Source: CAD feature listing. Evaluate the final solid. Frame: model axes, mm. A direction names the side the tool comes from. Round coordinates to 2 decimals unless told otherwise and drop trailing zeros. Write each loop counter-clockwise with the first axis right and the second up, starting at its lowest first coordinate (ties: lowest second). Pieces come first, ordered by that corner, then holes.
from build123d import *

# Parameters (mm, degrees)
F0_W           = 101.6
F0_H           = 203.2
F1_DEPTH       = 25.4
F2_W           = 22.9419407606
F2_H           = 22.7780664682
F2_W_2         = 22.94193331
F2_W_3         = 22.9362
F2_H_2         = 22.6314
F3_DEPTH       = 70.612
F4_W           = 50.8
F4_H           = 203.2
F5_DEPTH       = 9.525
F6_W           = 101.6606390476
F6_H           = 50.6004877388
F7_DEPTH       = 9.525
F8_W           = 50.696041435
F8_H           = 203.55078578
F9_DEPTH       = 9.525
F10_W          = 101.6
F10_H          = 50.8
F11_DEPTH      = 0.762
F11_DEPTH_BACK = 25.4
F12_DEPTH      = 25.4
F13_R          = 12.6564144883
F14_DEPTH      = 33.02


with BuildPart() as f1:
    # F0 (on Front) → F1 (new body)
    with BuildSketch(Plane.XZ):
        Rectangle(F0_W, F0_H)
    extrude(amount=F1_DEPTH)

    # F2 (on face) → F3 (join)
    with BuildSketch(Plane.XZ.offset(25.4)):
        with Locations((39.3290296197, 90.2109667659)):
            Rectangle(F2_W, F2_H)
        with Locations((-39.329033345, 90.2109667659)):
            Rectangle(F2_W_2, F2_H)
        with Locations((-39.3319, -89.9565626328)):
            Rectangle(F2_W_3, F2_H_2)
        with Locations((39.3319, -90.2023647373)):
            Rectangle(F2_W_3, F2_H_2)
    extrude(amount=F3_DEPTH)

    # F4 (on face) → F5 (join)
    with BuildSketch(Plane.YZ.offset(50.8)):
        Rectangle(F4_W, F4_H)
    extrude(amount=F5_DEPTH)

    # F6 (on face) → F7 (join)
    with BuildSketch(Plane.XY.offset(101.6)):
        Rectangle(F6_W, F6_H)
    extrude(amount=F7_DEPTH)

    # F8 (on face) → F9 (join)
    with BuildSketch(Plane(origin=(-50.8, 0, 0), x_dir=(0, -1, 0), z_dir=(-1, 0, 0))):
        Rectangle(F8_W, F8_H)
    extrude(amount=F9_DEPTH)

    # F10 (on face) → F11 (join, two sides)
    with BuildSketch(Plane(origin=(0, 0, -101.6), x_dir=(1, 0, 0), z_dir=(0, 0, -1))) as f11_sk:
        Rectangle(F10_W, F10_H)
    extrude(amount=F11_DEPTH)
    extrude(f11_sk.sketch, amount=-F11_DEPTH_BACK)

    # F2 (on face) → F12 (join)
    with BuildSketch(Plane.XZ.offset(25.4)):
        with Locations((39.3290296197, 90.2109667659)):
            Rectangle(F2_W, F2_H)
        with Locations((-39.329033345, 90.2109667659)):
            Rectangle(F2_W_2, F2_H)
        with Locations((-39.3319, -89.9565626328)):
            Rectangle(F2_W_3, F2_H_2)
        with Locations((39.3319, -90.2023647373)):
            Rectangle(F2_W_3, F2_H_2)
    extrude(amount=F12_DEPTH)

    # F13 (on face) → F14 (join)
    with BuildSketch(Plane.XZ.offset(25.4)):
        Circle(F13_R)
    extrude(amount=-F14_DEPTH)


solid = f1.part
1) Section query B-B on z = 0. Return the cut outline in (x, y) (3 decimals).
Taken from the geometry:
outline: (-60.325, -25.348) - (-50.8, -25.348) - (-50.8, -25.4) - (60.325, -25.4) - (60.325, 25.4) - (50.8, 25.4) - (50.8, 0) - (12.656, 0) - (12.656, 7.62) - (-12.656, 7.62) - (-12.656, 0) - (-50.8, 0) - (-50.8, 25.348) - (-60.325, 25.348) - close
2) Pull-direction query (X, two-part tool) for faces 1 (the face through (-50.83, 0, 106)), 2 (the face through (50.8, -60, -90)), 3 (the face through (-1, 13, 101.6)); classes: released by +X, released by -X, zero draft, split by the parting line, or undercut.
Taken from the geometry:
face 1: released by -X
face 2: released by +X
face 3: undercut
3) Section query A-A on y = -75.5. Return the cut outline in (x, z).
Taken from the geometry:
outline: (-50.8, -101.27) - (-27.86, -101.27) - (-27.86, -78.64) - (-50.8, -78.64) - close; (-50.8, 78.82) - (-27.86, 78.82) - (-27.86, 101.6) - (-50.8, 101.6) - close; (27.86, -101.52) - (50.8, -101.52) - (50.8, -78.89) - (27.86, -78.89) - close; (27.86, 78.82) - (50.8, 78.82) - (50.8, 101.6) - (27.86, 101.6) - close
4) Material intervals for line 1 (X direction, y = 8, z = 67.5) (3 decimals); line 2 (Z direction, x = -47.5, y = -63); line 3 (Z direction, x = 32, y = -60), sorted ascending.
Taken from the geometry:
line 1: x = -60.325 to -50.8, 50.8 to 60.325
line 2: z = -101.27 to -78.64, 78.82 to 101.6
line 3: z = -101.52 to -78.89, 78.82 to 101.6
5) Contact query for flat-ended pins moving along their axis: P1, Ø12.5, axis at x = 2.5, z = 0.5, coming from the +Y side; P2, Ø4, axis at y = -77.5, z = 85, coming from the +X side; P3, Ø2, axis at x = 42.5, z = -53.5, coming from the -Y side. Output: stop coordinate, or through.
Taken from the geometry:
P1: stops at y = 7.62
P2: stops at x = 50.8
P3: stops at y = -25.4
6) Section query C-C on x = 23. Return the cut outline in (y, z) (3 decimals).
Taken from the geometry:
outline: (-25.4, -102.362) - (25.4, -102.362) - (25.4, -76.2) - (0, -76.2) - (0, 101.6) - (25.3, 101.6) - (25.3, 111.125) - (-25.3, 111.125) - (-25.3, 101.6) - (-25.4, 101.6) - close
7) Section query D-D on z = -22.5. Return the cut outline in (x, y) (3 decimals), then the cut area to 3 significant figures.
Taken from the geometry:
outline: (-60.325, -25.348) - (-50.8, -25.348) - (-50.8, -25.4) - (60.325, -25.4) - (60.325, 25.4) - (50.8, 25.4) - (50.8, 0) - (-50.8, 0) - (-50.8, 25.348) - (-60.325, 25.348) - close
area: 3,550 mm2
8) Reachability of faces 4 (the face through (39, -60, 78.822)), 5 (the face through (-55, -25.348, -1)), 6 (the face through (50.83, 0, 106)), 7 (the face through (27.864, -60, -90)) from +Z, -Z, +X, -X, +Y, -Y: full face, straight path, thin tool, end or side. Return the list, or none.
Taken from the geometry:
face 4: +X, -X, -Y
face 5: +Z, -Z, -X, -Y
face 6: +Z, +X, +Y, -Y
face 7: +Z, -Z, -Y
